Check sheet for the modelled part. Datum: model origin and axes. Units: mm. A direction names the side the tool comes from. Round coordinates to 2 decimals unless told otherwise and drop trailing zeros. Write each loop counter-clockwise with the first axis right and the second up, starting at its lowest first coordinate (ties: lowest second). Pieces come first, ordered by that corner, then holes.
Item 1: Go/stop test with flat-tipped pins: pin 1 Ø3.5 at (y, z) = (24, 19) entering from +X; pin 2 Ø2 at (x, z) = (103, -9.5) entering from -Y; pin 3 Ø3 at (y, z) = (13.5, -10) entering from -X; pin 4 Ø5.5 at (y, z) = (22, 15.5) entering from -X. Record where each tip stops, or that it passes through.
Item 2: Material ranges on line 1 (Y direction, x = 30, z = 17.5); line 2 (Y direction, x = 0, z = -18); line 3 (Y direction, x = 99, z = -6), recorded low to high.
Item 3: Cross-section at D-D on y = 18.5. Enter the section's corners in (x, z).
Item 4: Release check for a two-part mould opening along X. For faces 1 (the flat face through (79.908, 7.395, 17.594)), 2 (the cylindrical face through (26, 24, -18)), 3 (the cylindrical face through (12.497, 7.93, 0.275)), 4 (the flat face through (-10, 8, -12.5)) record: +X half, -X half, draft (parallel to the pull), parting line (faces both ways), or undercut.
Item 5: Cross-section at B-B on z = 0. Enter the section's corners in (x, y), plus the area to 3 significant figures.
Item 6: Cross-section at C-C on x = -9.5. Enter the section's corners in (y, z), plus the area to 3 significant figures.
Item 7: Cross-section at A-A on x = 30. Enter the section's corners in (y, z).
Item 8: Tool access check on faces 5 (the flat face through (13, 3, 0)), 6 (the flat face through (40, 24, -18)), 7 (the flat face through (-10, 8, 12.5)), 8 (the flat face through (30, 21, 12.5)), 9 (the flat face through (-20, 9, -17)). Record the directions out of +Z, -Z, +X, -X, +Y, -Y that give a thin tool (end or side, any length) a straight path to the whole face; none if there is none.
from build123d import *

# Parameters (mm, degrees)
DODANIE_WYCI_GNI_CIE1_DEPTH = 15
WYTNIJ_WYCI_GNI_CIE1_DEPTH  = 46
SZKIC3_R                    = 5
DODANIE_WYCI_GNI_CIE2_DEPTH = 10
ZAOKR_GLENIE1_R             = 5
ZAOKR_GLENIE1_OF_LUSTRO1_R  = 5
SFAZOWANIE1_SIZE            = 2
OTW_R_GWINTOWANY_M121_D     = 10.2


with BuildPart() as part:
    # Szkic1 → Dodanie-wyciągnięcie1 (new body)
    with BuildSketch(Plane(origin=(0, 0, 0), x_dir=(1, 0, 0), z_dir=(0, 1, 0))):
        with BuildLine():
            Line((-20, 12.5), (-20, 22.5))
            Line((-20, 22.5), (45, 22.5))
            Line((45, 22.5), (113.85281653, 12.823367693))
            ThreePointArc((113.85281653, 12.823367693), (125, 0), (113.85281653, -12.823367693))
            Line((113.85281653, -12.823367693), (45, -22.5))
            Line((45, -22.5), (-20, -22.5))
            Line((-20, -22.5), (-20, -12.5))
            Line((-20, -12.5), (0, -12.5))
            ThreePointArc((0, -12.5), (12.5, 0), (0, 12.5))
            Line((0, 12.5), (-20, 12.5))
        make_face()
    extrude(amount=DODANIE_WYCI_GNI_CIE1_DEPTH)

    # Szkic2 → Wytnij-wyciągnięcie1 (cut, through all)
    with BuildSketch(Plane.XY.offset(22.5)):
        with BuildLine():
            Line((-20, 3), (15, 3))
            ThreePointArc((15, 3), (17.121320344, 2.121320344), (18, 0))
            Line((18, 0), (-20, 0))
            Line((-20, 0), (-20, 3))
        make_face()
    extrude(amount=-WYTNIJ_WYCI_GNI_CIE1_DEPTH, mode=Mode.SUBTRACT)

    # Szkic3 → Dodanie-wyciągnięcie2 (add)
    with BuildSketch(Plane.XY.offset(22.5)):
        with BuildLine():
            Line((20, 15), (20, 27))
            ThreePointArc((20, 27), (30, 37), (40, 27))
            Line((40, 27), (40, 15))
            Line((40, 15), (20, 15))
        make_face()
        with Locations((30, 27)):
            Circle(SZKIC3_R, mode=Mode.SUBTRACT)
    dodanie_wyci_gni_cie2 = extrude(amount=-DODANIE_WYCI_GNI_CIE2_DEPTH)

    # Zaokrąglenie1
    zaokr_glenie1_edges = [part.edges().sort_by_distance(p)[0] for p in [
        (40, 15, 17.5),
        (20, 15, 17.5),
    ]]
    fillet(zaokr_glenie1_edges, radius=ZAOKR_GLENIE1_R)

    # Lustro1: Dodanie-wyciągnięcie2 across plane
    add(dodanie_wyci_gni_cie2.mirror(Plane.XY))

    # Zaokrąglenie1 of Lustro1
    zaokr_glenie1_of_lustro1_edges = [part.edges().sort_by_distance(p)[0] for p in [
        (40, 15, -17.5),
        (20, 15, -17.5),
    ]]
    fillet(zaokr_glenie1_of_lustro1_edges, radius=ZAOKR_GLENIE1_OF_LUSTRO1_R)

    # Sfazowanie1
    sfazowanie1_edges = [part.edges().sort_by_distance(p)[0] for p in [
        (-10, 15, 12.5),
        (-10, 15, -12.5),
        (12.5, 15, 0),
    ]]
    chamfer(sfazowanie1_edges, length=SFAZOWANIE1_SIZE)

    # Otwór gwintowany M121 (through all)
    with Locations(Plane(origin=(0, 15, 0), x_dir=(1, 0, 0), z_dir=(0, 1, 0))):
        with Locations((112.050609731, 0)):
            Hole(OTW_R_GWINTOWANY_M121_D / 2)


solid = part.part
Response values:
1. pin 1: stops at x = 40
1. pin 2: stops at y = 0
1. pin 3: stops at x = 5.1
1. pin 4: stops at x = 19.94
2. line 1: y = 0 to 22, 32 to 37
2. line 2: y = 3 to 15
2. line 3: y = 0 to 15
3. outline: (19.77, -22.5) - (40.23, -22.5) - (40.23, -12.5) - (19.77, -12.5) - close; (19.77, 12.5) - (40.23, 12.5) - (40.23, 22.5) - (19.77, 22.5) - close
4. face 1: +X half
4. face 2: undercut
4. face 3: -X half
4. face 4: draft
5. outline: (12.5, 3) - (15, 3) arc R3 cw to (18, 0) - (106.95, 0) - (106.95, 15) - (14.5, 15) - (12.5, 13) - close; (117.15, 0) - (125, 0) - (125, 15) - (117.15, 15) - close
5. area: 1,520 mm2
6. outline: (3, -22.5) - (15, -22.5) - (15, -14.5) - (13, -12.5) - (3, -12.5) - close; (3, 12.5) - (13, 12.5) - (15, 14.5) - (15, 22.5) - (3, 22.5) - close
6. area: 236 mm2
7. outline: (0, -22.5) - (22, -22.5) - (22, -12.5) - (15, -12.5) - (15, 12.5) - (22, 12.5) - (22, 22.5) - (0, 22.5) - close; (32, -22.5) - (37, -22.5) - (37, -12.5) - (32, -12.5) - close; (32, 12.5) - (37, 12.5) - (37, 22.5) - (32, 22.5) - close
8. face 5: +Z, -Z, -X, -Y
8. face 6: +Z, -Z, +X, +Y
8. face 7: -X, +Y, -Y
8. face 8: +X, -X, +Y
8. face 9: +Z, -Z, -X, +Y, -Y
